Read the model definition and answer for the solid it produces. Units are mm, in the model's axes. A direction names the side the tool comes from. Coordinates: 2 decimals unless noted, no trailing zeros. Order: outer loops, then holes, each group sorted by start corner. A loop starts at its lowest first (then second) coordinate and runs counter-clockwise, first axis right, second up. Notation, with made-up numbers: (-37, 67.5) -> (17, 67.5) arc R15 ccw to (17, 86.5) -> close; hole circle Ø8 at (29.25, 32.25). An arc over 180 degrees is marked (long way). Answer as a JSON object with one key per item and string values. Group by question number.
1) Section A-A on y = 10 is taken. Determine the outline of the cut face in (x, z) (3 decimals).
2) Consider L1, parallel to X at y = 20.5, z = 12.5; L2, parallel to X at y = 25, z = -0.75; L3, parallel to Z at x = 24, y = 29.5 (3 decimals). Determine where each line is inside the solid, lowest interval first.
3) A tool of negligible diameter and unlimited length cuts with its end or side. For faces 5 (the flat face through (14, 26, 3.175)), 6 (the flat face through (-7, 30.48, -1)), 7 (the flat face through (2, 30, 13.386)), 8 (the flat face through (48, 17.78, -1)), from which of +Z, -Z, +X, -X, +Y, -Y can it reach the whole face along a straight path? Write none if from no direction.
4) Section C-C on x = 19 is taken. Determine the outline of the cut face in (y, z) (3 decimals).
5) Determine the mould class of faces 1 (the flat face through (-6, 23, 1.905)), 2 (the cylindrical face through (26.975, 25.002, -0.044)), 3 (the flat face through (40.132, 24, 7)), 4 (the flat face through (20, 43.18, 2)) for opening direction X: released by +X, released by -X, zero draft, split by the parting line, or undercut.
6) Given pin 1 (4 mm diameter, centred on y = 35, z = 7, fed in from -X); pin 2 (1.7 mm diameter, centred on x = 12.446, y = 25.654, fed in from +Z); pin 3 (8.5 mm diameter, centred on y = 24, z = 6.5, fed in from -X); pin 4 (5 mm diameter, centred on x = 26.5, y = 24.5, fed in from +Z) (3 decimals), each flat-ended and moving along its own axis, determine where each tip first touches the part or whether it passes through.
7) Section B-B on z = 0.75 is taken. Count the separate pieces of the cut face and the enclosed holes in it, and give its area (3 significant figures).
8) Section D-D on x = -10 is taken. Determine the outline of the cut face in (y, z) (3 decimals), and give its area (3 significant figures).
Autodesk Inventor part; units mm, degrees
ref_plane "YZ Plane" through (0, 0, 0) normal (1, 0, 0) x (0, 1, 0)
ref_plane "XZ Plane" through (0, 0, 0) normal (0, 1, 0) x (-1, 0, 0)
ref_plane "XY Plane" through (0, 0, 0) normal (0, 0, 1) x (1, 0, 0)
sketch "Sketch1" plane through (0, 0, 0) normal (0, 0, 1) x (1, 0, 0)
  line L0 (0, 0) -> (40.132, 0)
  line L1 (40.132, 0) -> (40.132, 48.26)
  line L2 (40.132, 48.26) -> (0, 48.26)
  line L3 (0, 48.26) -> (0, 0)
  line L4 (3.556, 44.704) -> (36.576, 44.704) construction
  line L5 (36.576, 44.704) -> (36.576, 1.524) construction
  line L6 (36.576, 1.524) -> (3.556, 1.524) construction
  line L7 (3.556, 1.524) -> (3.556, 44.704) construction
  line L8 (37.592, 1.016) -> (37.592, 45.72)
  line L9 (37.592, 45.72) -> (2.54, 45.72)
  line L10 (2.54, 45.72) -> (2.54, 1.016)
  line L11 (2.54, 1.016) -> (37.592, 1.016) construction
  line L12 (2.54, 1.016) -> (2.54, 0)
  line L13 (37.592, 1.016) -> (37.592, 0)
  line L14 (12.446, 25.654) -> (27.686, 25.654)
  point P0 (20.066, 48.26)
  point P1 (20.066, 44.704)
  point P2 (3.556, 23.114)
  point P3 (0, 24.13)
  point P4 (20.066, 25.654)
  dimension "d2" = 33.02
  dimension "d3" = 43.18
  dimension "d4" = 1.524
  dimension "d8" = 2.54
  dimension "d9" = 1.016
  dimension "d14" = 15.24
  dimension "d15" = 19.05
  dimension "d34" = 1.016
  dimension "d35" = 1.016
extrude "Extrusion1" add sketch "Sketch1" against normal blind 3.175
sketch "Sketch2" plane through (0, 0, 0) normal (0, 0, 1) x (1, 0, 0)
  line L0 (2.54, 1.016) -> (2.54, 0)
  line L1 (0, 48.26) -> (0, 0)
  line L2 (2.54, 45.72) -> (2.54, 1.016)
  line L3 (37.592, 45.72) -> (2.54, 45.72)
  line L4 (40.132, 48.26) -> (0, 48.26)
  line L5 (40.132, 0) -> (40.132, 48.26)
  line L6 (37.592, 1.016) -> (37.592, 0)
  line L7 (37.592, 1.016) -> (37.592, 45.72)
  line L8 (0, 0) -> (2.54, 0)
  line L9 (37.592, 0) -> (40.132, 0)
extrude "Extrusion2" add sketch "Sketch2" along normal blind 13.3856
sketch "Sketch3" plane through (0, 0, 0) normal (0, 0, 1) x (1, 0, 0)
  line L0 (2.54, 1.016) -> (37.592, 1.016)
  line L1 (2.54, 0) -> (37.592, 0)
  line L2 (2.54, 0) -> (2.54, 45.72)
  line L3 (37.592, 45.72) -> (37.592, 0)
  point P0 (0, 0)
extrude "Extrusion3" add sketch "Sketch3" along normal blind 4.775
sketch "Sketch4" plane through (0, 0, 0) normal (0, 0, 1) x (1, 0, 0)
  circle A0 centre (12.446, 25.654) radius 3.175
  circle A1 centre (27.686, 25.654) radius 3.175
  circle A2 centre (12.446, 25.654) radius 0.9652
  circle A3 centre (27.686, 25.654) radius 0.9652
  point P0 (0, 0)
  dimension "d16" = 6.35
  dimension "d18" = 1.9304
extrude "Extrusion4" add sketch "Sketch4" along normal blind 3.175
extrude "Extrusion8" cut sketch "Sketch4" against normal through all contours A2 | A3
sketch "Sketch5" plane through (0, 0, 0) normal (0, 0, 1) x (1, 0, 0)
  circle A0 centre (12.446, 25.654) radius 3.175 construction
  circle A1 centre (27.686, 25.654) radius 3.175 construction
  line L0 (2.54, 1.016) -> (37.592, 1.016) construction
  line L1 (37.592, 1.016) -> (37.592, 45.72) construction
  line L2 (37.592, 45.72) -> (2.54, 45.72) construction
  line L3 (2.54, 45.72) -> (2.54, 1.016) construction
  line L4 (3.556, 44.704) -> (36.576, 44.704) construction
  line L5 (3.556, 1.524) -> (3.556, 44.704) construction
  line L6 (36.576, 44.704) -> (36.576, 1.524) construction
  line L7 (36.576, 1.524) -> (3.556, 1.524) construction
  line L8 (2.54, 1.016) -> (37.592, 1.016)
  line L9 (37.592, 1.016) -> (37.592, 3.048)
  line L10 (37.592, 3.048) -> (2.54, 3.048)
  line L11 (2.54, 3.048) -> (2.54, 1.016)
  line L12 (2.54, 45.72) -> (37.592, 45.72)
  line L13 (37.592, 45.72) -> (37.592, 43.18)
  line L14 (37.592, 43.18) -> (2.54, 43.18)
  line L15 (2.54, 43.18) -> (2.54, 45.72)
  point P0 (0, 0)
  dimension "d21" = 1.524
  dimension "d25" = 1.524
extrude "Extrusion5" add sketch "Sketch5" along normal blind 3.175
sketch "Sketch6" plane through (0, 0, 4.775) normal (0, 0, 1) x (1, 0, 0)
  line L0 (40.132, 0) -> (0, 0) construction
  line L1 (4.826, 0) -> (2.54, 0)
  line L2 (2.54, 0) -> (2.54, 1.016)
  line L3 (2.54, 1.016) -> (4.826, 1.016)
  line L4 (4.826, 1.016) -> (4.826, 0)
  line L5 (2.54, 0) -> (2.54, 45.72)
  line L6 (37.592, 1.016) -> (2.54, 1.016) construction
  line L7 (35.306, 0) -> (37.592, 0)
  line L8 (37.592, 0) -> (37.592, 1.016)
  line L9 (37.592, 1.016) -> (35.306, 1.016)
  line L10 (35.306, 1.016) -> (35.306, 0)
  dimension "d26" = 2.286
  dimension "d27" = 2.286
extrude "Extrusion6" add sketch "Sketch6" along normal up to surface (8.6106 mm away)
fillet "Fillet1" radius 2.286 2 edges at (37.592, 1.016, 8.2803) (2.54, 1.016, 8.2803)
chamfer "Chamfer2" distance 1.524 angle 45 2 edges at (9.271, 25.654, 0) (24.511, 25.654, 0)
fillet "Fillet2" radius 3.175 4 edges at (0, 0, 5.1053) (40.132, 0, 5.1053) (40.132, 48.26, 5.1053) (0, 48.26, 5.1053)
sketch "Sketch7" plane through (0, 0, -3.175) normal (0, 0, -1) x (-1, 0, 0)
  circle A0 centre (8.509, 24.13) radius 2.5527
  line L0 (-3.175, 48.26) -> (-36.957, 48.26) construction
  line L1 (-40.132, 45.085) -> (-40.132, 3.175) construction
  line L2 (-36.957, 0) -> (-3.175, 0) construction
  line L3 (0, 3.175) -> (0, 45.085) construction
  line L4 (-40.132, 48.26) -> (0, 48.26) construction
  line L5 (-20.066, 48.26) -> (-20.066, 0) construction
  arc A1 (0, 36.83) -> (6.35, 30.48) centre (6.35, 36.83) ccw
  arc A2 (6.35, 17.78) -> (0, 11.43) centre (6.35, 11.43) ccw
  line L6 (6.35, 30.48) -> (8.509, 30.48)
  arc A3 (8.509, 17.78) -> (8.509, 30.48) centre (8.509, 24.13) ccw
  line L7 (8.509, 17.78) -> (6.35, 17.78)
  line L8 (0, 36.83) -> (0, 11.43)
  line L9 (0, 0) -> (0, 48.26)
  circle A4 centre (-48.641, 24.13) radius 2.5527
  arc A5 (-46.482, 30.48) -> (-40.132, 36.83) centre (-46.482, 36.83) ccw
  arc A6 (-40.132, 11.43) -> (-46.482, 17.78) centre (-46.482, 11.43) ccw
  line L10 (-46.482, 30.48) -> (-48.641, 30.48)
  arc A7 (-48.641, 30.48) -> (-48.641, 17.78) centre (-48.641, 24.13) ccw
  line L11 (-48.641, 17.78) -> (-46.482, 17.78)
  line L12 (-40.132, 36.83) -> (-40.132, 11.43)
  arc A8 (0, 45.085) -> (-3.175, 48.26) centre (-3.175, 45.085) ccw
  arc A9 (-36.957, 48.26) -> (-40.132, 45.085) centre (-36.957, 45.085) ccw
  arc A10 (-40.132, 3.175) -> (-36.957, 0) centre (-36.957, 3.175) ccw
  arc A11 (-3.175, 0) -> (0, 3.175) centre (-3.175, 3.175) ccw
  point P0 (-3.175, 48.26)
  point P1 (0, 24.13)
  point P2 (-40.132, 24.13)
  dimension "d40" = 5.1054
  dimension "d41" = 6.35
  dimension "d43" = 6.35
  dimension "d44" = 57.15
extrude "Extrusion7" add sketch "Sketch7" against normal blind 5.08
fillet "Fillet3" radius 3.175 2 edges at (40.132, 24.13, 1.905) (0, 24.13, 1.905)
equation "\"d12\" = BoardOffset + PCBThickness"
equation "\"d19\" = BoardOffset"
equation "\"d23\" = BoardOffset"
equation "\"d27\" = d26"
equation "\"d28\" = BoardOffset"
equation "\"PCBThickness\" = 1.6"
equation "\"BoardOffset\" = 3.175"
properties part number "TOF Case P1"
Worked answers:
{
 "1": {"outline": "(0, -3.175) -> (40.132, -3.175) -> (40.132, 13.386) -> (37.592, 13.386) -> (37.592, 0) -> (2.54, 0) -> (2.54, 13.386) -> (0, 13.386) -> close"},
 "2": {"L1": "x = 0 to 2.54, 37.59 to 40.13", "L2": "x = -14.8 to -10.91, -6.11 to 11.74, 13.16 to 26.98, 28.4 to 46.24, 51.04 to 54.93", "L3": "z = -3.175 to 0"},
 "3": {"face 5": "+Z", "face 6": "+Z, -Z, -X, +Y", "face 7": "+Z, +X, -X, +Y, -Y", "face 8": "+Z, -Z, +X, -Y"},
 "4": {"outline": "(0, -3.175) -> (48.26, -3.175) -> (48.26, 13.386) -> (45.72, 13.386) -> (45.72, 3.175) -> (43.18, 3.175) -> (43.18, 0) -> (3.048, 0) -> (3.048, 3.175) -> (1.016, 3.175) -> (1.016, 4.775) -> (0, 4.775) -> close"},
 "5": {"face 1": "zero draft", "face 2": "undercut", "face 3": "released by +X", "face 4": "undercut"},
 "6": {"pin 1": "stops at x = 0", "pin 2": "passes through", "pin 3": "stops at x = -1.74", "pin 4": "stops at z = 3.175"},
 "7": {"separate pieces": "3", "enclosed holes": "5", "area": "950 mm²"},
 "8": {"outline": "(17.958, -3.175) -> (22.058, -3.175) -> (22.058, 1.905) -> (17.958, 1.905) -> close; (26.202, -3.175) -> (30.302, -3.175) -> (30.302, 1.905) -> (26.202, 1.905) -> close", "area": "41.7 mm²"}
}
